The drawing under review shows one solid part. Ordinate dimensions are in mm from its lowest x, y, z. A direction names the side the tool comes from. Coordinates: 2 decimals unless noted, no trailing zeros. Loops run counter-clockwise (first coordinate to the right, second up) from the corner with the lowest first, then second, coordinate; pieces in that order, holes last. Notation, with made-up numbers: M 54,-35.5 L 79,-35.5 A21 cw 79,-23.5 Z; hole C -32,-27.5 d1. An arc over 180 degrees is marked long. Answer as CSV lines item,"result". Start each with the question number.
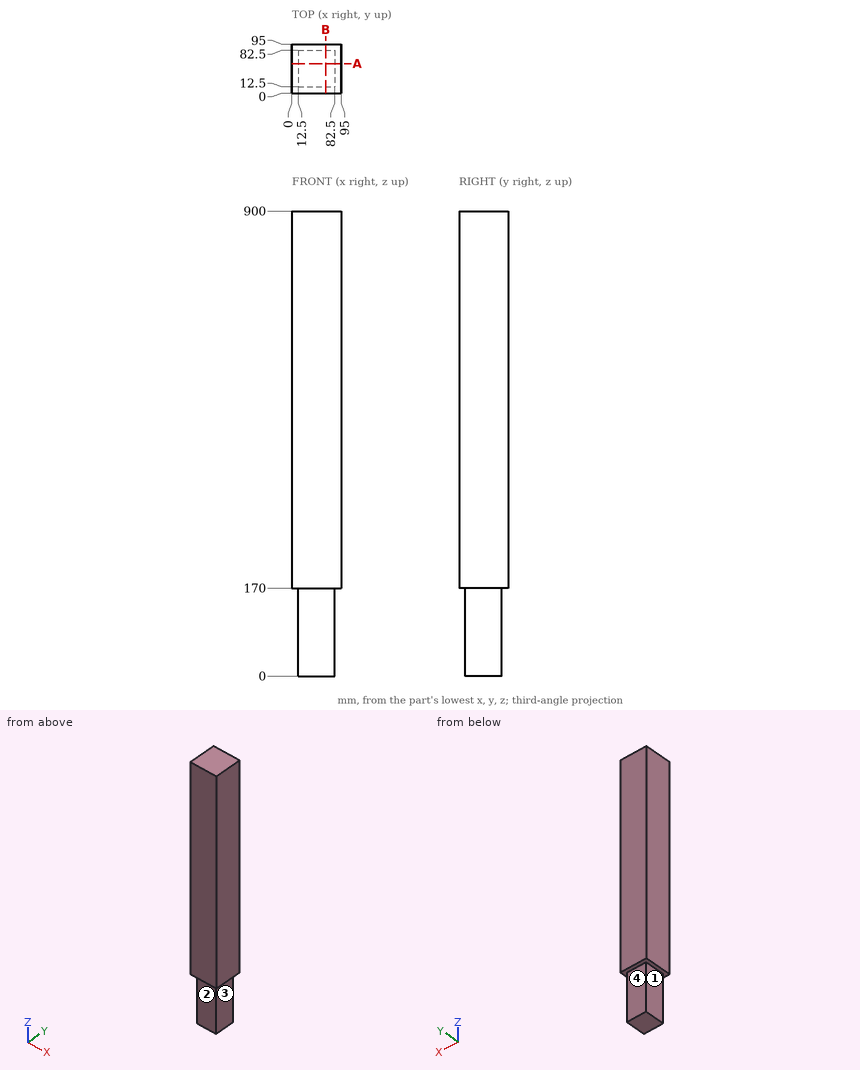
Item 1: For line 1 along Z through (x, y) = (7, 5.5); line 2 along Y through (x, z) = (43, 169), list the stretches that pass through material, from the lowest coordinate up. Write a range as from..to.
Item 2: For pin 1 (21 mm diameter, centred on y = 36.5, z = 71, fed in from +X); pin 2 (5 mm diameter, centred on x = 82, y = 43, fed in from -Z), all flat-tipped, find the tip position at first contact; note any pin that passes through.
Item 3: Add section A-A (y = 57). Give the boundary of the cut face in (x, z).
Item 4: For the marked faces 1, 2, 3 and 4, list the 3-axis set-ups (+Z, -Z, +X, -X, +Y, -Y) from which the entire face can be reached by the end or side of a thin tool; tool diameter is ignored.
Response:
1,line 1,"170..900"
1,line 2,"12.5..82.5"
2,pin 1,"x = 82.5"
2,pin 2,"z = 0"
3,outline,"M 0,170 L 12.5,170 L 12.5,0 L 82.5,0 L 82.5,170 L 95,170 L 95,900 L 0,900 Z"
4,face 1,"-Z, -X, +Y, -Y"
4,face 2,"-Z, +X, -X, -Y"
4,face 3,"-Z, +X, +Y, -Y"
4,face 4,"-Z, +X, -X, +Y"
